Part model, mm, in its own coordinate system. A direction names the side the tool comes from. Coordinates: 2 decimals unless noted, no trailing zeros. Loops run counter-clockwise (first coordinate to the right, second up) from the corner with the lowest first, then second, coordinate; pieces in that order, holes last. Notation, with made-up numbers: M 80,-12.5 L 137,-12.5 A19 ccw 137,3.5 Z; hole C 31,2 d10. An arc over 180 degrees is marked long. Use a Markdown table: item, result. Add a question column.
1) Wall check: probe 1 along Y at (x, z) = (0, 6.5); probe 2 along Y at (x, z) = (0, 12); probe 3 along Z at (x, y) = (26, 12.5). Give the ranges that are in metal, low to high. Write a range as from..to.
2) Tool access for faces 4 (the cylindrical face through (22.355, -9.269, 8.944)), 5 (the cylindrical face through (30.236, 9.522, 6.563)), 6 (the flat face through (0, -7, 0)): list every direction of +Z, -Z, +X, -X, +Y, -Y with a clear straight run to the whole face (end or side of a thin tool).
3) Band-saw the part on C-C (z = 7). List the corners of the cut face in (x, y).
4) Pull direction Y, two halves, no side cores. Call faces 1 (the flat face through (0, 6, 5)), 2 (the flat face through (-24, -21, 11)), 3 (the cylindrical face through (30.713, 9.672, 1.014)): released by +Y, released by -Y, zero draft, split by the parting line, or undercut.
5) Band-saw the part on D-D (x = 13). List the corners of the cut face in (y, z), plus the area to 3 significant figures.
6) Band-saw the part on A-A (x = 0). List the corners of the cut face in (y, z), plus the area to 4 significant figures.
7) Pin check, flat tips, straight feed: pin 1 Ø1.5 at (x, z) = (-19.5, 4.5) entering from +Y; pin 2 Ø4 at (x, y) = (0, -17.5) entering from +Z; pin 3 Ø1 at (x, z) = (10, 8.5) entering from +Y. Stop position of each tip, or through.
from build123d import *

# Parameters (mm, degrees)
F0_W     = 5
F0_H     = 10
F3_R     = 1.75
F4_DEPTH = 40


with BuildPart() as f1:
    # F0 (on Front) → F1 (revolve)
    with BuildSketch(Plane.XZ):
        with Locations((2.5, 10)):
            Rectangle(F0_W, F0_H)
        Polygon((0, 5), (0, 0), (32.2, 0), (32.2, 2), (31.7, 2), (31.7, 11), (32.2, 11), (32.2, 13), (24.2, 13), (24.2, 5), (5, 5), align=None)
    revolve(axis=Axis((0, 0, 10), (0, 0, 1)))

    # F3 (on face) → F4 (cut)
    with BuildSketch(Plane.XY.offset(15)):
        Circle(F3_R)
    extrude(amount=-F4_DEPTH, mode=Mode.SUBTRACT)


solid = f1.part
Entries:
| question | item | result |
|---|---|---|
| 1 | probe 1 | -31.7..-24.2, -5..-1.75, 1.75..5, 24.2..31.7 |
| 1 | probe 2 | -32.2..-24.2, -5..-1.75, 1.75..5, 24.2..32.2 |
| 1 | probe 3 | 0..13 |
| 2 | face 4 | +Z |
| 2 | face 5 | none |
| 2 | face 6 | -Z, +X, -X, +Y, -Y |
| 3 | outline | C 0,0 d63.4; C 0,0 d10; hole C 0,0 d48.4; hole C 0,0 d3.5 |
| 4 | face 1 | undercut |
| 4 | face 2 | zero draft |
| 4 | face 3 | split by the parting line |
| 5 | outline | M -29.46,0 L 29.46,0 L 29.46,2 L 28.91,2 L 28.91,11 L 29.46,11 L 29.46,13 L 20.41,13 L 20.41,5 L -20.41,5 L -20.41,13 L -29.46,13 L -29.46,11 L -28.91,11 L -28.91,2 L -29.46,2 Z |
| 5 | area | 429 mm2 |
| 6 | outline | M -32.2,0 L -1.75,0 L -1.75,15 L -5,15 L -5,5 L -24.2,5 L -24.2,13 L -32.2,13 L -32.2,11 L -31.7,11 L -31.7,2 L -32.2,2 Z; M 1.75,0 L 32.2,0 L 32.2,2 L 31.7,2 L 31.7,11 L 32.2,11 L 32.2,13 L 24.2,13 L 24.2,5 L 5,5 L 5,15 L 1.75,15 Z |
| 6 | area | 488.5 mm2 |
| 7 | pin 1 | y = 25.56 |
| 7 | pin 2 | z = 5 |
| 7 | pin 3 | y = 30.24 |
